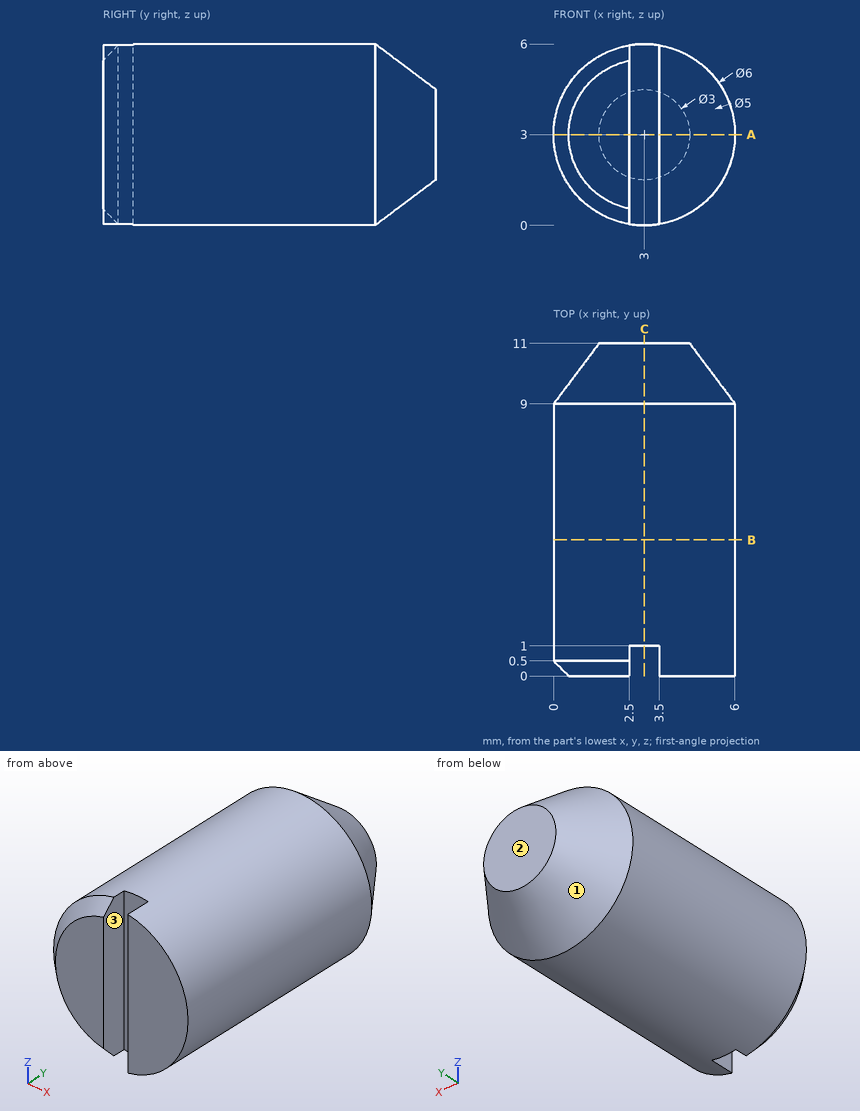
Study the drawing (mm; zero at the part's minimum x, y, z) and answer. Give positions to 0.01 mm unless a question says otherwise; leave off trailing zeros. Write each loop counter-clockwise with the first axis right and the second up, starting at its lowest first coordinate (ties: lowest second). Pieces come first, ordered by that corner, then holes. Notation, with made-up numbers: (42, 80.5) - (93, 80.5) arc R25 ccw to (93, 106.5) - close; hole circle Ø11 at (29.25, 23). An arc over 180 degrees is marked (long way). Use a Markdown table: item, result.
1. Find the intervals of material crossed by probe 1 along X at (y, z) = (0.75, 5.7); probe 2 along X at (y, z) = (8, 1.85); probe 3 along Y at (x, z) = (2.7, 3.1), in increasing order. Write a range as from..to.
Values follow:
| item | result |
|---|---|
| probe 1 | x = 1.69..2.5, 3.5..4.31 |
| probe 2 | x = 0.23..5.77 |
| probe 3 | y = 1..11 |
2. Section B-B on y = 4.5 is taken. Write down the section's boundary in (x, z).
Values follow:
| item | result |
|---|---|
| outline | circle Ø6 at (3, 3) |
3. For a pull along X with two mould halves and no side action, classify the marked faces 1, 2 and 3 as released by +X, released by -X, zero draft, split by the parting line, or undercut.
Values follow:
| item | result |
|---|---|
| face 1 | split by the parting line |
| face 2 | zero draft |
| face 3 | undercut |
4. Section A-A on z = 3 is taken. Write down the section's boundary in (x, y).
Values follow:
| item | result |
|---|---|
| outline | (0, 0.5) - (0.5, 0) - (2.5, 0) - (2.5, 1) - (3.5, 1) - (3.5, 0) - (6, 0) - (6, 9) - (4.5, 11) - (1.5, 11) - (0, 9) - close |
5. Section C-C on x = 3 is taken. Write down the section's boundary in (y, z).
Values follow:
| item | result |
|---|---|
| outline | (1, 0) - (9, 0) - (11, 1.5) - (11, 4.5) - (9, 6) - (1, 6) - close |
